Check sheet for the modelled part. Datum: model origin and axes. Units: mm. Face numbers are marked on the shaded views. A direction names the side the tool comes from. Round coordinates to 2 decimals unless told otherwise and drop trailing zeros. Order: outer loops, then holes, each group sorted by start corner. A loop starts at its lowest first (then second) coordinate and runs counter-clockwise, first axis right, second up.
(1) Mould release check, pull along X, two halves, no side actions. Record for the marked faces 4, 5 and 6: released by +X, released by -X, zero draft, split by the parting line, or undercut.
(2) Sectioned sample at C-C, the plane z = 15. Enter the section's corners in (x, y), and give its area (3 significant figures).
(3) Sectioned sample at D-D, the plane x = -17. Enter the section's corners in (y, z), and give its area (3 significant figures).
(4) Depth check by flat-ended pin: pin 1 (10 mm diameter, centred on y = -1.5, z = 13.5, fed in from +X); pin 2 (4 mm diameter, centred on x = -9.5, y = 4.5, fed in from +Z); pin 3 (12 mm diameter, centred on x = 6, z = 33.5, fed in from -Y). Enter the tip coordinate at first touch or a pass-through.
(5) Thickness scan on probe 1 along Z at (x, y) = (1, -12); probe 2 along X at (y, z) = (-4.5, 7); probe 3 along X at (y, z) = (-15, 20) (3 decimals). Record the ranges inside material, lowest first.
(6) Sectioned sample at B-B, the plane y = 0. Count the separate pieces of the cut face and the enclosed holes in it, and give its area (3 significant figures).
(7) Sectioned sample at A-A, the plane x = 0. Enter the section's corners in (y, z), and give its area (3 significant figures).
(8) Tool access check on the marked faces 1, 2 and 3. Record the directions out of +Z, -Z, +X, -X, +Y, -Y that give a thin tool (end or side, any length) a straight path to the whole face; none if there is none.
```python
from build123d import *

# Parameters (mm, degrees)
SKETCH_1_R      = 24
EXTRUDE_1_DEPTH = 2
SKETCH_2_R      = 3
EXTRUDE_2_DEPTH = 17
SKETCH_3_R      = 24
EXTRUDE_3_DEPTH = 2
SKETCH_4_R      = 3.25
EXTRUDE_4_DEPTH = 16.5


with BuildPart() as part:
    # 草图1 → 凸台-拉伸1 (new body)
    with BuildSketch(Plane.XY):
        Circle(SKETCH_1_R)
        with BuildLine():
            Line((-11.739632055, -14.042831804), (-10.057601798, -9.597641998))
            ThreePointArc((-10.057601798, -9.597641998), (-9.353754198, -8.978695741), (-8.446592755, -9.214394762))
            ThreePointArc((-8.446592755, -9.214394762), (0, -12.5), (8.446592755, -9.214394762))
            ThreePointArc((8.446592755, -9.214394762), (9.353754198, -8.978695741), (10.057601798, -9.597641998))
            Line((10.057601798, -9.597641998), (11.739632055, -14.042831804))
            ThreePointArc((11.739632055, -14.042831804), (11.764677024, -14.675613965), (11.404592123, -15.196554824))
            ThreePointArc((11.404592123, -15.196554824), (0, -19), (-11.404592123, -15.196554824))
            ThreePointArc((-11.404592123, -15.196554824), (-11.764677024, -14.675613965), (-11.739632055, -14.042831804))
        make_face(mode=Mode.SUBTRACT)
        with BuildLine():
            Line((-18.03126511, -3.145403689), (-13.340602686, -3.91131766))
            ThreePointArc((-13.340602686, -3.91131766), (-12.452655704, -3.611240886), (-12.203196322, -2.70776652))
            ThreePointArc((-12.203196322, -2.70776652), (-10.825317547, 6.25), (-3.756603567, 11.922161282))
            ThreePointArc((-3.756603567, 11.922161282), (-3.098901506, 12.589936627), (-3.283000887, 13.508959657))
            Line((-3.283000887, 13.508959657), (-6.291633055, 17.188235493))
            ThreePointArc((-6.291633055, 17.188235493), (-6.827115998, 17.526316153), (-7.458306466, 17.47494391))
            ThreePointArc((-7.458306466, 17.47494391), (-16.454482672, 9.5), (-18.862898589, -2.278389086))
            ThreePointArc((-18.862898589, -2.278389086), (-18.591793022, -2.850702188), (-18.03126511, -3.145403689))
        make_face(mode=Mode.SUBTRACT)
        with BuildLine():
            Line((6.291633055, 17.188235493), (3.283000887, 13.508959657))
            ThreePointArc((3.283000887, 13.508959657), (3.098901506, 12.589936627), (3.756603567, 11.922161282))
            ThreePointArc((3.756603567, 11.922161282), (10.825317547, 6.25), (12.203196322, -2.70776652))
            ThreePointArc((12.203196322, -2.70776652), (12.452655704, -3.611240886), (13.340602686, -3.91131766))
            Line((13.340602686, -3.91131766), (18.03126511, -3.145403689))
            ThreePointArc((18.03126511, -3.145403689), (18.591793022, -2.850702188), (18.862898589, -2.278389086))
            ThreePointArc((18.862898589, -2.278389086), (16.454482672, 9.5), (7.458306466, 17.47494391))
            ThreePointArc((7.458306466, 17.47494391), (6.827115998, 17.526316153), (6.291633055, 17.188235493))
        make_face(mode=Mode.SUBTRACT)
    extrude(amount=EXTRUDE_1_DEPTH)

    # 草图2 → 凸台-拉伸2 (add)
    with BuildSketch(Plane.XY.offset(2)):
        Circle(SKETCH_2_R)
        with Locations((0, 8.5)):
            Circle(SKETCH_2_R)
        with Locations((7.361215932, -4.25)):
            Circle(SKETCH_2_R)
        with Locations((-7.361215932, -4.25)):
            Circle(SKETCH_2_R)
    extrude(amount=EXTRUDE_2_DEPTH)

    # 草图3 → 凸台-拉伸3 (add)
    with BuildSketch(Plane.XY.offset(19)):
        Circle(SKETCH_3_R)
        with BuildLine():
            Line((-10.057601798, -9.597641998), (-11.739632055, -14.042831804))
            ThreePointArc((-11.739632055, -14.042831804), (-11.764677024, -14.675613965), (-11.404592123, -15.196554824))
            ThreePointArc((-11.404592123, -15.196554824), (0, -19), (11.404592123, -15.196554824))
            ThreePointArc((11.404592123, -15.196554824), (11.764677024, -14.675613965), (11.739632055, -14.042831804))
            Line((11.739632055, -14.042831804), (10.057601798, -9.597641998))
            ThreePointArc((10.057601798, -9.597641998), (9.353754198, -8.978695741), (8.446592755, -9.214394762))
            ThreePointArc((8.446592755, -9.214394762), (0, -12.5), (-8.446592755, -9.214394762))
            ThreePointArc((-8.446592755, -9.214394762), (-9.353754198, -8.978695741), (-10.057601798, -9.597641998))
        make_face(mode=Mode.SUBTRACT)
        with BuildLine():
            Line((6.291633055, 17.188235493), (3.283000887, 13.508959657))
            ThreePointArc((3.283000887, 13.508959657), (3.098901506, 12.589936627), (3.756603567, 11.922161282))
            ThreePointArc((3.756603567, 11.922161282), (10.825317547, 6.25), (12.203196322, -2.70776652))
            ThreePointArc((12.203196322, -2.70776652), (12.452655704, -3.611240886), (13.340602686, -3.91131766))
            Line((13.340602686, -3.91131766), (18.03126511, -3.145403689))
            ThreePointArc((18.03126511, -3.145403689), (18.591793022, -2.850702188), (18.862898589, -2.278389086))
            ThreePointArc((18.862898589, -2.278389086), (16.454482672, 9.5), (7.458306466, 17.47494391))
            ThreePointArc((7.458306466, 17.47494391), (6.827115998, 17.526316153), (6.291633055, 17.188235493))
        make_face(mode=Mode.SUBTRACT)
        with BuildLine():
            Line((-3.283000887, 13.508959657), (-6.291633055, 17.188235493))
            ThreePointArc((-6.291633055, 17.188235493), (-6.827115998, 17.526316153), (-7.458306466, 17.47494391))
            ThreePointArc((-7.458306466, 17.47494391), (-16.454482672, 9.5), (-18.862898589, -2.278389086))
            ThreePointArc((-18.862898589, -2.278389086), (-18.591793022, -2.850702188), (-18.03126511, -3.145403689))
            Line((-18.03126511, -3.145403689), (-13.340602686, -3.91131766))
            ThreePointArc((-13.340602686, -3.91131766), (-12.452655704, -3.611240886), (-12.203196322, -2.70776652))
            ThreePointArc((-12.203196322, -2.70776652), (-10.825317547, 6.25), (-3.756603567, 11.922161282))
            ThreePointArc((-3.756603567, 11.922161282), (-3.098901506, 12.589936627), (-3.283000887, 13.508959657))
        make_face(mode=Mode.SUBTRACT)
    extrude(amount=EXTRUDE_3_DEPTH)

    # 草图4 → 凸台-拉伸4 (add)
    with BuildSketch(Plane.XY.offset(21)):
        Circle(SKETCH_4_R)
    extrude(amount=EXTRUDE_4_DEPTH)


solid = part.part
```
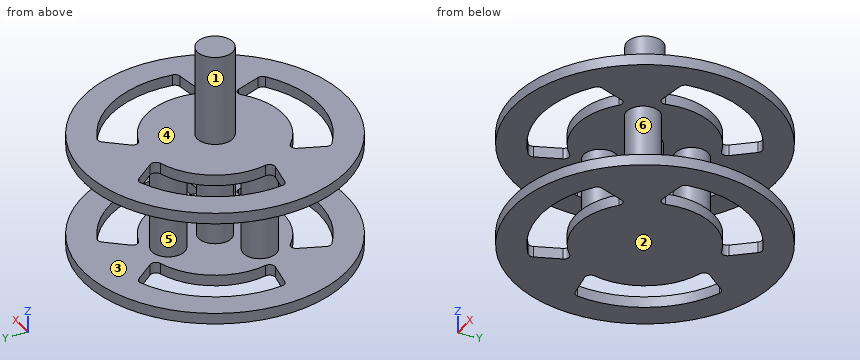
Derived:
1. face 4: zero draft
1. face 5: split by the parting line
1. face 6: undercut
2. outline: circle Ø6 at (-7.36, -4.25); circle Ø6 at (0, 0); circle Ø6 at (0, 8.5); circle Ø6 at (7.36, -4.25)
2. area: 113 mm2
3. outline: (-16.94, 0) - (-3.31, 0) - (-3.31, 2) - (-16.94, 2) - close; (-16.94, 19) - (-3.31, 19) - (-3.31, 21) - (-16.94, 21) - close; (8.49, 0) - (16.94, 0) - (16.94, 2) - (8.49, 2) - close; (8.49, 19) - (16.94, 19) - (16.94, 21) - (8.49, 21) - close
3. area: 88.3 mm2
4. pin 1: stops at x = 10.36
4. pin 2: stops at z = 21
4. pin 3: stops at y = -3.25
5. probe 1: z = 0 to 2, 19 to 21
5. probe 2: x = -10.35 to -4.37, 4.37 to 10.35
5. probe 3: x = -18.735 to -11.602, 11.602 to 18.735
6. separate pieces: 5
6. enclosed holes: 0
6. area: 349 mm2
7. outline: (-24, 0) - (-19, 0) - (-19, 2) - (-24, 2) - close; (-24, 19) - (-19, 19) - (-19, 21) - (-24, 21) - close; (-12.5, 0) - (24, 0) - (24, 2) - (11.5, 2) - (11.5, 19) - (24, 19) - (24, 21) - (3.25, 21) - (3.25, 37.5) - (-3.25, 37.5) - (-3.25, 21) - (-12.5, 21) - (-12.5, 19) - (-3, 19) - (-3, 2) - (-12.5, 2) - close; hole (3, 2) - (5.5, 2) - (5.5, 19) - (3, 19) - close
7. area: 477 mm2
8. face 1: +Z
8. face 2: -Z, +X, -X, +Y, -Y
8. face 3: none
